Geometry: see drawing. Coordinates: mm, zero at the bounding-box minimum. Round coordinates to 2 decimals unless told otherwise and drop trailing zeros. Order: outer loops, then holes, each group sorted by start corner. A loop starts at its lowest first (then second) coordinate and runs counter-clockwise, first axis right, second up. Notation, with made-up numbers: (-2, 11) -> (45, 11) arc R24 ccw to (45, 36) -> close; hole circle Ø11 at (54, -31.5). An arc over 180 degrees is marked (long way). Use a Markdown table: item, result.
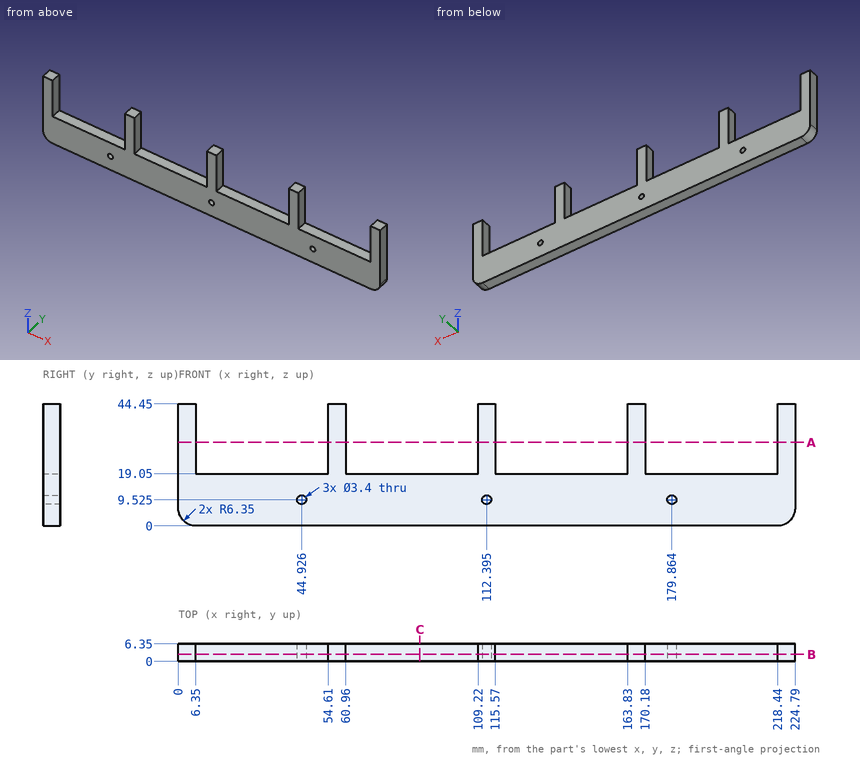
1) Contact query for flat-ended pins moving along their axis: P1, Ø1.9, axis at x = 88, y = 3.5, coming from the +Z side; P2, Ø3, axis at x = 112.395, z = 9.525, coming from the +Y side. Output: stop coordinate, or through.
Answer key:
| item | result |
|---|---|
| P1 | stops at z = 19.05 |
| P2 | passes through |
2) Cut plane C-C on x = 88. Return loops of the section in (y, z), and give its area (3 significant figures).
Answer key:
| item | result |
|---|---|
| outline | (0, 0) -> (6.35, 0) -> (6.35, 19.05) -> (0, 19.05) -> close |
| area | 121 mm^2 |
3) Ray query, probe 1 along X at (y, z) = (1, 35.5); probe 2 along Z at (x, y) = (159, 6). Return the intervals inside material, ascending.
Answer key:
| item | result |
|---|---|
| probe 1 | x = 0 to 6.35, 54.61 to 60.96, 109.22 to 115.57, 163.83 to 170.18, 218.44 to 224.79 |
| probe 2 | z = 0 to 19.05 |
4) Cut plane A-A on z = 30.5. Return loops of the section in (x, y), and give its area (3 significant figures).
Answer key:
| item | result |
|---|---|
| outline | (0, 0) -> (6.35, 0) -> (6.35, 6.35) -> (0, 6.35) -> close; (54.61, 0) -> (60.96, 0) -> (60.96, 6.35) -> (54.61, 6.35) -> close; (109.22, 0) -> (115.57, 0) -> (115.57, 6.35) -> (109.22, 6.35) -> close; (163.83, 0) -> (170.18, 0) -> (170.18, 6.35) -> (163.83, 6.35) -> close; (218.44, 0) -> (224.79, 0) -> (224.79, 6.35) -> (218.44, 6.35) -> close |
| area | 202 mm^2 |
5) Cut plane B-B on y = 2.5. State how many separate pieces and enclosed holes the cut face has, and give its area (3 significant figures).
Answer key:
| item | result |
|---|---|
| separate pieces | 1 |
| enclosed holes | 3 |
| area | 5,040 mm^2 |
